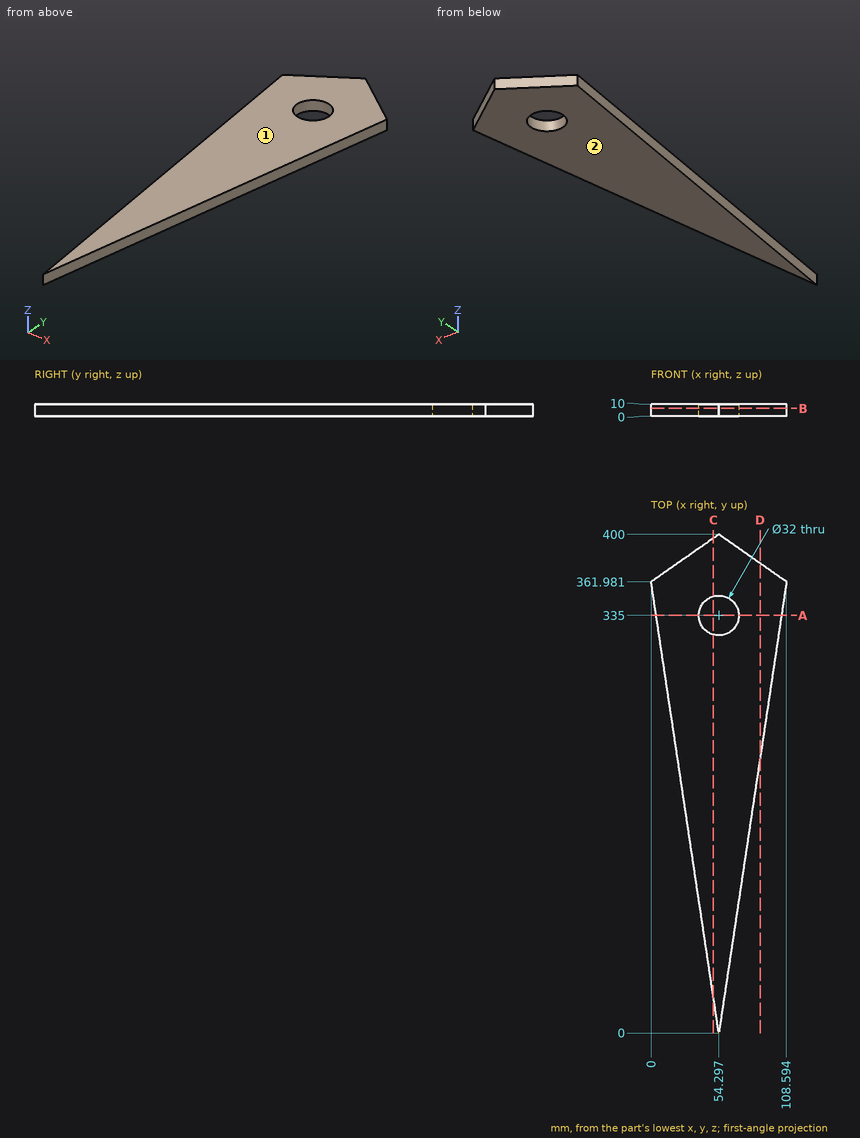
Design review of the part shown in the three views and the two pictorial views. Dimensions are in mm from the part's minimum x, y and z. Give positions to 0.01 mm unless a question says otherwise; leave off trailing zeros. Write each loop counter-clockwise with the first axis right and the second up, starting at its lowest first coordinate (ties: lowest second). Pieces come first, ordered by that corner, then holes. Notation, with made-up numbers: M 45,56 L 66,56 A7 ccw 66,67 Z; hole C 49,35.25 d2. An arc over 180 degrees is marked long. One line per item, written item: value.
1) For P1, Ø6, axis at y = 113, z = 4.5, coming from the +X side; P2, Ø1, axis at x = 51, z = 5, coming from the +Y side; P3, Ø1.5, axis at y = 136.5, z = 2, coming from the +X side (1 decimal); P4, Ø10, axis at x = 52.5, y = 255.5, coming from the -Z side, all flat-tipped, find the tip position at first contact; note any pin that passes through.
Results are:
P1: stops at x = 71.7
P2: stops at y = 398.04
P3: stops at x = 74.9
P4: stops at z = 0
2) Take a section at D-D, the plane x = 87.5. Write out the cut boundary in (y, z).
Results are:
outline: M 221.35,0 L 376.75,0 L 376.75,10 L 221.35,10 Z
3) Take a section at B-B, the plane z = 6.5. Write out the cut boundary in (x, y).
Results are:
outline: M 0,361.98 L 54.3,0 L 108.59,361.98 L 54.3,400 Z; hole C 54.3,335 d32
4) For line 1 (X direction, y = 344.5, z = 7.5); line 2 (X direction, y = 212.5, z = 1.75); line 3 (X direction, y = 59, z = 5.5), list the stretches that pass through material, from the lowest coordinate up. Write a range as from..to.
Results are:
line 1: x = 2.62..41.42, 67.17..105.97
line 2: x = 22.42..86.17
line 3: x = 45.45..63.15
5) Take a section at A-A, the plane y = 335. Write out the cut boundary in (x, z), then the cut area to 3 significant figures.
Results are:
outline: M 4.05,0 L 38.3,0 L 38.3,10 L 4.05,10 Z; M 70.3,0 L 104.55,0 L 104.55,10 L 70.3,10 Z
area: 685 mm²
6) The part is to be moulded in two halves that separate along Z. For the marked faces 1 and 2, say which applies: +Z half, -Z half, draft (parallel to the pull), parting line (faces both ways), or undercut.
Results are:
face 1: +Z half
face 2: -Z half
7) Take a section at C-C, the plane x = 50. Write out the cut boundary in (y, z).
Results are:
outline: M 28.65,0 L 319.59,0 L 319.59,10 L 28.65,10 Z; M 350.41,0 L 396.99,0 L 396.99,10 L 350.41,10 Z
